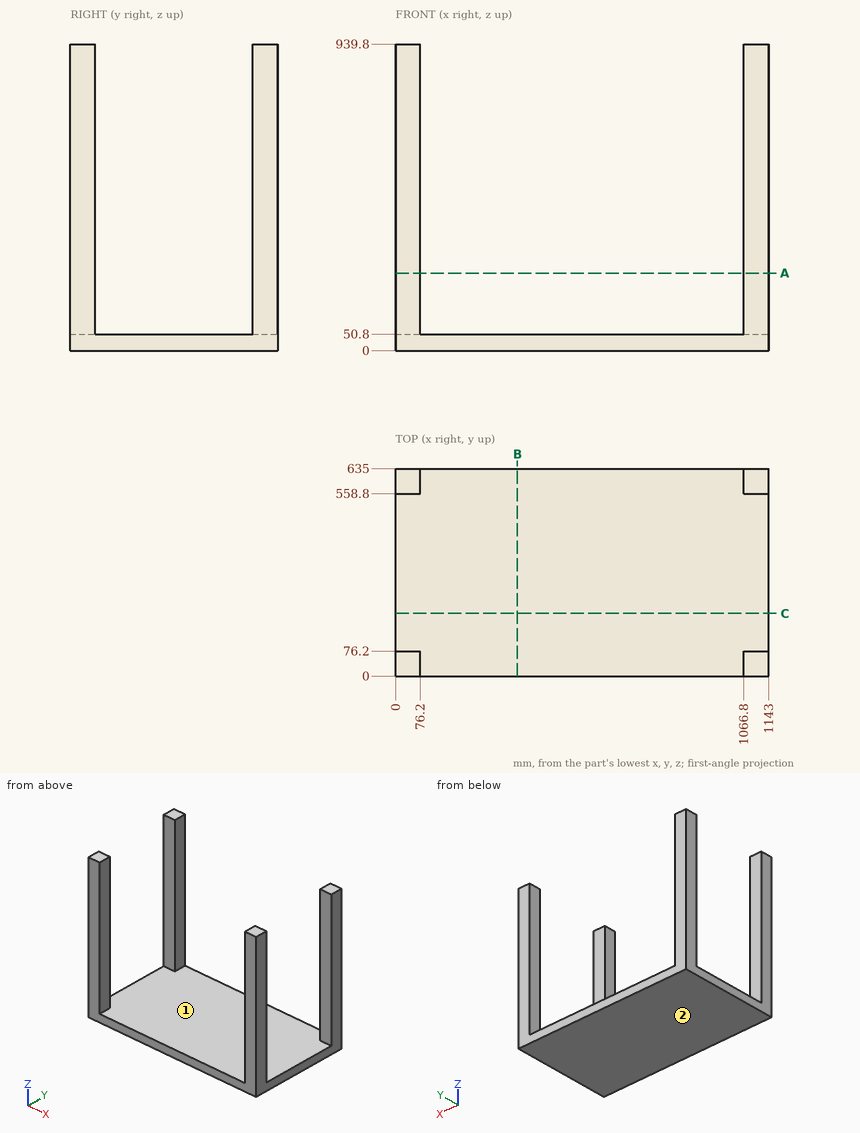
Print and shaded views of the part. All mm, measured from the part's lowest x, y and z. Coordinates: 2 decimals unless noted, no trailing zeros. Loops run counter-clockwise (first coordinate to the right, second up) from the corner with the lowest first, then second, coordinate; pieces in that order, holes last. Notation, with made-up numbers: (-3.75, 72) - (13.25, 72) arc R29 ccw to (13.25, 106) - close; hole circle Ø11 at (25.25, 76.25). An arc over 180 degrees is marked (long way). Use one line per item in the form item = value. Start each with the question number.
1) Flat gauge pin, fed straight in: pin 1 (1 mm diameter, centred on x = 359.5, y = 328.5, fed in from +Z). Where does the tip first touch, or does it go through?
2) Band-saw the part on A-A (z = 238). Give the cut face in (x, y).
3) Band-saw the part on B-B (x = 373). Give the cut face in (y, z), and give its area (3 significant figures).
4) Drill centre lines: L1, parallel to X at y = 37, z = 610; L2, parallel to Z at x = 805, y = 394; L3, parallel to Y at x = 1091.5, z = 875.5. Where is each one in solid material? Low to high. Write a range as from..to.
5) Two-plate mould, pull along X, no slides. Class the marked faces 1 and 2: +X half, -X half, draft (parallel to the pull), parting line (faces both ways), or undercut.
6) Band-saw the part on C-C (y = 192). Give the cut face in (x, z), and give its area (3 significant figures).
Check values:
q1.pin_1 = 50.8
q2.outline = (0, 0) - (76.2, 0) - (76.2, 76.2) - (0, 76.2) - close; (0, 558.8) - (76.2, 558.8) - (76.2, 635) - (0, 635) - close; (1066.8, 0) - (1143, 0) - (1143, 76.2) - (1066.8, 76.2) - close; (1066.8, 558.8) - (1143, 558.8) - (1143, 635) - (1066.8, 635) - close
q3.outline = (0, 0) - (635, 0) - (635, 50.8) - (0, 50.8) - close
q3.area = 32,300 mm2
q4.L1 = 0..76.2, 1066.8..1143
q4.L2 = 0..50.8
q4.L3 = 0..76.2, 558.8..635
q5.face_1 = undercut
q5.face_2 = draft
q6.outline = (0, 0) - (1143, 0) - (1143, 50.8) - (0, 50.8) - close
q6.area = 58,100 mm2
